Source: CAD feature listing. Evaluate the final solid. Frame: model axes, mm. A direction names the side the tool comes from. Give positions to 0.01 mm unless a question says otherwise; leave off trailing zeros. Loops run counter-clockwise (first coordinate to the right, second up) from the corner with the lowest first, then second, coordinate; pieces in that order, holes last. Notation, with made-up numbers: (52.5, -40) -> (105.5, -40) arc R32 cw to (105.5, -14) -> close; hole circle Ø2 at (75.5, 13.25). An arc over 180 degrees is marked (long way). Return JSON: item names as keys, results as strings. Group by question number.
(1) Ray query, line 1 (X direction, y = 0, z = -2); line 2 (X direction, y = 1, z = 54.5). Return the intervals inside material, ascending. Write a range as from..to.
(2) Access query for faces 4 (the face through (-29.97, 1.32, 29.85)), 5 (the face through (0, 0, 0)), 6 (the face through (0, 0, 5)). Directions: +Z, -Z, +X, -X, +Y, -Y. A direction counts if a zero-diameter tool reaches every point of the face in a straight line with its end or side. Return the directions, or none.
(3) Draft query along Y for faces 1 (the face through (23.846, -7.509, -4.93)), 2 (the face through (-11, -17, -10)), 3 (the face through (-5.85, -26.36, 33.11)). Return one class per face: released by +Y, released by -Y, zero draft, split by the parting line, or undercut.
(4) Pin query (flat end, axial travel): pin 1 (10 mm diameter, centred on y = 12.5, z = 26, fed in from +X); pin 2 (1.5 mm diameter, centred on x = -15, y = 24, fed in from -Z); pin 3 (5 mm diameter, centred on y = -8.5, z = 11.5, fed in from -X). Return the tip coordinate at first contact, or that it passes through.
(5) Cut plane C-C on z = 36. Return loops of the section in (x, y).
```python
from build123d import *

# Parameters (mm, degrees)
F0_R       = 30
F1_DEPTH   = 60
F2_R       = 27
F1_FACE1_R = 30
F3_DEPTH   = 55
F4_R       = 25
F5_DEPTH   = 10
F6_R       = 20
F7_DEPTH   = 10
F8_R       = 1.49999
F9_R       = 2
F10_R      = 2


# Not quite as in the source:
# - a fillet or chamfer is up to 0.001 mm smaller than in the source, because OpenCascade refuses the exact size


with BuildPart() as f1:
    # F0 (on Top) → F1 (new body)
    with BuildSketch(Plane.XY):
        Circle(F0_R)
    extrude(amount=F1_DEPTH)

    # F2 (on face) + F1_face1 (on face) → F3 (cut)
    with BuildSketch(Plane.XY.offset(60)):
        Circle(F2_R)
    with BuildSketch(Plane(origin=(0, 0, 0), x_dir=(1, 0, 0), z_dir=(0, 0, -1))):
        Circle(F1_FACE1_R)
    extrude(amount=-F3_DEPTH, dir=(0, 0, 1), mode=Mode.SUBTRACT)

    # F4 (on face) → F5 (join)
    with BuildSketch(Plane(origin=(0, 0, 0), x_dir=(1, 0, 0), z_dir=(0, 0, -1))):
        Circle(F4_R)
    extrude(amount=F5_DEPTH)

    # F6 (on face) → F7 (cut)
    with BuildSketch(Plane(origin=(0, 0, -10), x_dir=(1, 0, 0), z_dir=(0, 0, -1))):
        Circle(F6_R)
    extrude(amount=-F7_DEPTH, mode=Mode.SUBTRACT)

    # F8 (radius 1.5 in the source; OpenCascade refuses exactly that, so slightly less here)
    f8_edges = [f1.edges().sort_by_distance(p)[0] for p in [
        (-30, 0, 60),
        (-27, 0, 60),
    ]]
    fillet(f8_edges, radius=F8_R)

    # F9
    f9_edges = [f1.edges().sort_by_distance(p)[0] for p in [
        (-30, 0, 0),
    ]]
    fillet(f9_edges, radius=F9_R)

    # F10
    f10_edges = [f1.edges().sort_by_distance(p)[0] for p in [
        (-27, 0, 5),
    ]]
    fillet(f10_edges, radius=F10_R)


solid = f1.part
```
Answers:
{
 "1": {"line 1": "-25..-20, 20..25", "line 2": "-29.98..-26.98, 26.98..29.98"},
 "2": {"face 4": "+Z, -Z", "face 5": "-Z", "face 6": "+Z"},
 "3": {"face 1": "split by the parting line", "face 2": "zero draft", "face 3": "undercut"},
 "4": {"pin 1": "x = 29.05", "pin 2": "z = 0", "pin 3": "x = -29.39"},
 "5": {"outline": "circle Ø60 at (0, 0); hole circle Ø54 at (0, 0)"}
}
